Can you work these out from the model? Positions are in its coordinate system, mm. A direction names the side the tool comes from. Coordinates: 2 decimals unless noted, no trailing zeros. Order: outer loops, then holes, each group sorted by start corner. A loop starts at its lowest first (then second) coordinate and runs counter-clockwise, first axis right, second up. Notation, with made-up numbers: (68, 36.25) -> (93, 36.25) arc R24 ccw to (93, 66.25) -> close; hole circle Ø10 at (-23, 31). An arc over 180 degrees is marked (long way). Answer as CSV lines item,"result".
Autodesk Inventor part; units mm, degrees
ref_plane "YZ Plane" through (0, 0, 0) normal (1, 0, 0) x (0, 1, 0)
ref_plane "XZ Plane" through (0, 0, 0) normal (0, 1, 0) x (-1, 0, 0)
ref_plane "XY Plane" through (0, 0, 0) normal (0, 0, 1) x (1, 0, 0)
sketch "Sketch1" plane through (0, 0, 0) normal (0, 1, 0) x (-1, 0, 0)
  circle A0 centre (0, 0) radius 7.5
  line L0 (8.0698, 1.3309) -> (7.381, 1.3309)
  line L1 (7.381, -1.3309) -> (8.0698, -1.3309)
  line L2 (12.3774, -0.5735) -> (12.3774, -0.474)
  line L3 (12.3774, 1.3309) -> (7.5, 0) construction
  line L4 (7.5, 0) -> (12.3774, -1.3309) construction
  line L5 (11.8209, 0) -> (11.8209, 0.7484)
  arc A1 (11.8209, 0.7484) -> (7.381, 1.3309) centre (7.7254, -13.2556) ccw
  line L6 (7.5, 0) -> (12.3774, 0)
  line L7 (12.3774, -1.3309) -> (7.5, 0) construction
  line L8 (11.8209, 0) -> (11.8209, -0.7484)
  arc A2 (7.381, -1.3309) -> (11.8209, -0.7484) centre (7.7254, 13.2556) ccw
  arc A3 (5.7266, -4.8431) -> (9.863, -6.5586) centre (13.3182, 7.617) ccw
  arc A4 (10.6114, -5.2623) -> (7.0576, -2.5379) centre (0.0626, -15.3424) ccw
  line L9 (10.2372, -5.9105) -> (10.6114, -5.2623)
  line L10 (10.2372, -5.9105) -> (9.863, -6.5586)
  arc A5 (2.5379, -7.0576) -> (5.2623, -10.6114) centre (15.3424, -0.0626) ccw
  arc A6 (6.5586, -9.863) -> (4.8431, -5.7266) centre (-7.617, -13.3182) ccw
  line L11 (5.9105, -10.2372) -> (6.5586, -9.863)
  line L12 (5.9105, -10.2372) -> (5.2623, -10.6114)
  arc A7 (-1.3309, -7.381) -> (-0.7484, -11.8209) centre (13.2556, -7.7254) ccw
  arc A8 (0.7484, -11.8209) -> (1.3309, -7.381) centre (-13.2556, -7.7254) ccw
  line L13 (0, -11.8209) -> (0.7484, -11.8209)
  line L14 (0, -11.8209) -> (-0.7484, -11.8209)
  arc A9 (-4.8431, -5.7266) -> (-6.5586, -9.863) centre (7.617, -13.3182) ccw
  arc A10 (-5.2623, -10.6114) -> (-2.5379, -7.0576) centre (-15.3424, -0.0626) ccw
  line L15 (-5.9105, -10.2372) -> (-5.2623, -10.6114)
  line L16 (-5.9105, -10.2372) -> (-6.5586, -9.863)
  arc A11 (-7.0576, -2.5379) -> (-10.6114, -5.2623) centre (-0.0626, -15.3424) ccw
  arc A12 (-9.863, -6.5586) -> (-5.7266, -4.8431) centre (-13.3182, 7.617) ccw
  line L17 (-10.2372, -5.9105) -> (-9.863, -6.5586)
  line L18 (-10.2372, -5.9105) -> (-10.6114, -5.2623)
  arc A13 (-7.381, 1.3309) -> (-11.8209, 0.7484) centre (-7.7254, -13.2556) ccw
  arc A14 (-11.8209, -0.7484) -> (-7.381, -1.3309) centre (-7.7254, 13.2556) ccw
  line L19 (-11.8209, 0) -> (-11.8209, -0.7484)
  line L20 (-11.8209, 0) -> (-11.8209, 0.7484)
  arc A15 (-5.7266, 4.8431) -> (-9.863, 6.5586) centre (-13.3182, -7.617) ccw
  arc A16 (-10.6114, 5.2623) -> (-7.0576, 2.5379) centre (-0.0626, 15.3424) ccw
  line L21 (-10.2372, 5.9105) -> (-10.6114, 5.2623)
  line L22 (-10.2372, 5.9105) -> (-9.863, 6.5586)
  arc A17 (-2.5379, 7.0576) -> (-5.2623, 10.6114) centre (-15.3424, 0.0626) ccw
  arc A18 (-6.5586, 9.863) -> (-4.8431, 5.7266) centre (7.617, 13.3182) ccw
  line L23 (-5.9105, 10.2372) -> (-6.5586, 9.863)
  line L24 (-5.9105, 10.2372) -> (-5.2623, 10.6114)
  arc A19 (1.3309, 7.381) -> (0.7484, 11.8209) centre (-13.2556, 7.7254) ccw
  arc A20 (-0.7484, 11.8209) -> (-1.3309, 7.381) centre (13.2556, 7.7254) ccw
  line L25 (0, 11.8209) -> (-0.7484, 11.8209)
  line L26 (0, 11.8209) -> (0.7484, 11.8209)
  arc A21 (4.8431, 5.7266) -> (6.5586, 9.863) centre (-7.617, 13.3182) ccw
  arc A22 (5.2623, 10.6114) -> (2.5379, 7.0576) centre (15.3424, 0.0626) ccw
  line L27 (5.9105, 10.2372) -> (5.2623, 10.6114)
  line L28 (5.9105, 10.2372) -> (6.5586, 9.863)
  arc A23 (7.0576, 2.5379) -> (10.6114, 5.2623) centre (0.0626, 15.3424) ccw
  arc A24 (9.863, 6.5586) -> (5.7266, 4.8431) centre (13.3182, -7.617) ccw
  line L29 (10.2372, 5.9105) -> (9.863, 6.5586)
  line L30 (10.2372, 5.9105) -> (10.6114, 5.2623)
  line L31 (2.6226, -0.9781) -> (2.6226, -1.001)
  line L32 (2.6226, 1.001) -> (2.6226, 0.9781)
  line L33 (2.6226, 0.4136) -> (2.6226, 0.391)
  circle A25 centre (0, 0) radius 2.75
  point P0 (10.4324, -6.6853)
  point P1 (6.3232, -5.1875)
  point P2 (7.6541, -2.8823)
  point P3 (5.692, -11.0058)
  point P4 (2.8823, -7.6541)
  point P5 (5.1875, -6.3232)
  point P6 (-0.5735, -12.3774)
  point P7 (-1.3309, -8.0698)
  point P8 (1.3309, -8.0698)
  point P9 (-6.6853, -10.4324)
  point P10 (-5.1875, -6.3232)
  point P11 (-2.8823, -7.6541)
  point P12 (-11.0058, -5.692)
  point P13 (-7.6541, -2.8823)
  point P14 (-6.3232, -5.1875)
  point P15 (-12.3774, 0.5735)
  point P16 (-8.0698, 1.3309)
  point P17 (-8.0698, -1.3309)
  point P18 (-10.4324, 6.6853)
  point P19 (-6.3232, 5.1875)
  point P20 (-7.6541, 2.8823)
  point P21 (-5.692, 11.0058)
  point P22 (-2.8823, 7.6541)
  point P23 (-5.1875, 6.3232)
  point P24 (0.5735, 12.3774)
  point P25 (1.3309, 8.0698)
  point P26 (-1.3309, 8.0698)
  point P27 (6.6853, 10.4324)
  point P28 (5.1875, 6.3232)
  point P29 (2.8823, 7.6541)
  point P30 (11.0058, 5.692)
  point P31 (7.6541, 2.8823)
  point P32 (6.3232, 5.1875)
  point P33 (7.0576, -2.5379)
  point P34 (7.0576, 2.5379)
  point P35 (5.7266, 4.8431)
  point P36 (4.8431, 5.7266)
  point P37 (2.5379, 7.0576)
  point P38 (1.3309, 7.381)
  point P39 (-1.3309, 7.381)
  point P40 (-2.5379, 7.0576)
  point P41 (-4.8431, 5.7266)
  point P42 (-5.7266, 4.8431)
  point P43 (-7.0576, 2.5379)
  point P44 (-7.381, 1.3309)
  point P45 (-7.381, -1.3309)
  point P46 (-7.0576, -2.5379)
  point P47 (-5.7266, -4.8431)
  point P48 (-4.8431, -5.7266)
  point P49 (-2.5379, -7.0576)
  point P50 (-1.3309, -7.381)
  point P51 (1.3309, -7.381)
  point P52 (2.5379, -7.0576)
  point P53 (4.8431, -5.7266)
  dimension "d0" = 15
  dimension "d3" = 360
  dimension "d5" = 5.5
extrude "Extrusion1" add sketch "Sketch1" along normal blind 5 contours A0 | L6 L8 A2 L1 A0 | A0 L0 A1 L5 L6 | A0 A24 L29 L30 A23 | A4 L9 L10 A3 A0 | A0 A22 L27 L28 A21 | A6 L11 L12 A5 A0 | A0 A20 L25 L26 A19 | A8 L13 L14 A7 A0 | A0 A18 L23 L24 A17 | A10 L15 L16 A9 A0 | A0 A16 L21 L22 A15 | A12 L17 L18 A11 A0 | A0 A14 L19 L20 A13
sketch "Sketch2" plane through (0, 5, 0) normal (0, 1, 0) x (1, 0, 0)
  line L0 (-2.3094, 4) -> (2.3094, 4)
  line L1 (2.3094, 4) -> (4.6188, 0)
  line L2 (4.6188, 0) -> (2.3094, -4)
  line L3 (2.3094, -4) -> (-2.3094, -4)
  line L4 (-2.3094, -4) -> (-4.6188, 0)
  line L5 (-4.6188, 0) -> (-2.3094, 4)
  line L6 (0, 0) -> (-6.3613, 0)
  dimension "d8" = 8
extrude "Extrusion2" cut sketch "Sketch2" against normal blind 1
ref_plane "Work Plane1" through (0, 2.5, 0) normal (0, 1, 0) x (1, 0, 0)
mirror "Mirror1" about plane through (0, 2.5, 0) normal (0, 1, 0) of "Extrusion2"
properties part number "JointFixer"
Q1. If I drill on line 1 (Z direction, x = 0, y = 1.85); line 2 (Z direction, x = 0.5, y = 0.75), over which ranges is the centre line in solid material (lowest first)?
Solution:
line 1,"-11.82 to -2.75, 2.75 to 11.82"
line 2,"-11.82 to -4, 4 to 11.82"
Q2. Imagine slicing it at A-A (x = 0). List the corners of the cut face in (y, z) for me, and give its area (3 significant figures).
Solution:
outline,"(0, -11.82) -> (5, -11.82) -> (5, -4) -> (4, -4) -> (4, -2.75) -> (1, -2.75) -> (1, -4) -> (0, -4) -> close; (0, 4) -> (1, 4) -> (1, 2.75) -> (4, 2.75) -> (4, 4) -> (5, 4) -> (5, 11.82) -> (0, 11.82) -> close"
area,"85.7 mm2"
Q3. Which directions (+Z, -Z, +X, -X, +Y, -Y) give clear straight access to the entire face, cutting with the end or side of a thin tool? Please do faces 1 (the cylindrical face through (5.309, 2.465, 5.297)), 2 (the flat face through (3.448, 0.493, 2.028)), 3 (the cylindrical face through (-9.99, 2.46, -1.16)).
Solution:
face 1,"+Y, -Y"
face 2,"-Y"
face 3,"-X, +Y, -Y"
Q4. Imagine slicing it at C-C (z = -4.5). List the corners of the cut face in (x, y) for me, and give its area (3 significant figures).
Solution:
outline,"(-9.83, 0) -> (9.83, 0) -> (9.83, 5) -> (-9.83, 5) -> close"
area,"98.3 mm2"
Q5. Imagine slicing it at B-B (z = -7.75). List the corners of the cut face in (x, y) for me, and give its area (3 significant figures).
Solution:
outline,"(-5.87, 0) -> (-2.94, 0) -> (-2.94, 5) -> (-5.87, 5) -> close; (-1.33, 0) -> (1.33, 0) -> (1.33, 5) -> (-1.33, 5) -> close; (2.94, 0) -> (5.87, 0) -> (5.87, 5) -> (2.94, 5) -> close"
area,"42.6 mm2"
Q6. We'd pull the mould along X, two halves only. Please class faces 4 (the cylindrical face through (7.24, 2.46, -1.95)), 5 (the cylindrical face through (-3.78, 2.46, -8.96)), 6 (the cylindrical face through (1.215, 2.465, 9.592)), 7 (the flat face through (0, 2, 11.821)): pulls with the +X half, pulls with the -X half, needs draft (parallel to the pull), parting line crosses it, or undercut.
Solution:
face 4,"pulls with the +X half"
face 5,"undercut"
face 6,"undercut"
face 7,"needs draft"
Q7. For P1, Ø0.8, axis at x = 1, y = 0.5, coming from the -Z side; P2, Ø2, axis at x = -3.5, y = 1, coming from the +Z side; P3, Ø6.5, axis at x = 0, z = 0, coming from the +Y side; P4, Ø3, axis at y = 1, z = 8.5, coming from the -X side, each with a flat end and sliding along its axis, tell me the tip position at first contact or that it passes through.
Solution:
P1,"z = -11.82"
P2,"z = 9.83"
P3,"y = 4"
P4,"x = -6.56"
